Job drawing, mm, ordinate dimensions from the low corner. One solid piece. Give positions to 0.01 mm unless a question says otherwise; leave off trailing zeros. Order: outer loops, then holes, each group sorted by start corner. A loop starts at its lowest first (then second) coordinate and runs counter-clockwise, first axis right, second up. Notation, with made-up numbers: (5.5, 87.25) - (60.5, 87.25) arc R30 cw to (60.5, 126.25) - close; hole circle Ø4 at (62.5, 32.5). An arc over 180 degrees is marked (long way). One line per item, written item: value.
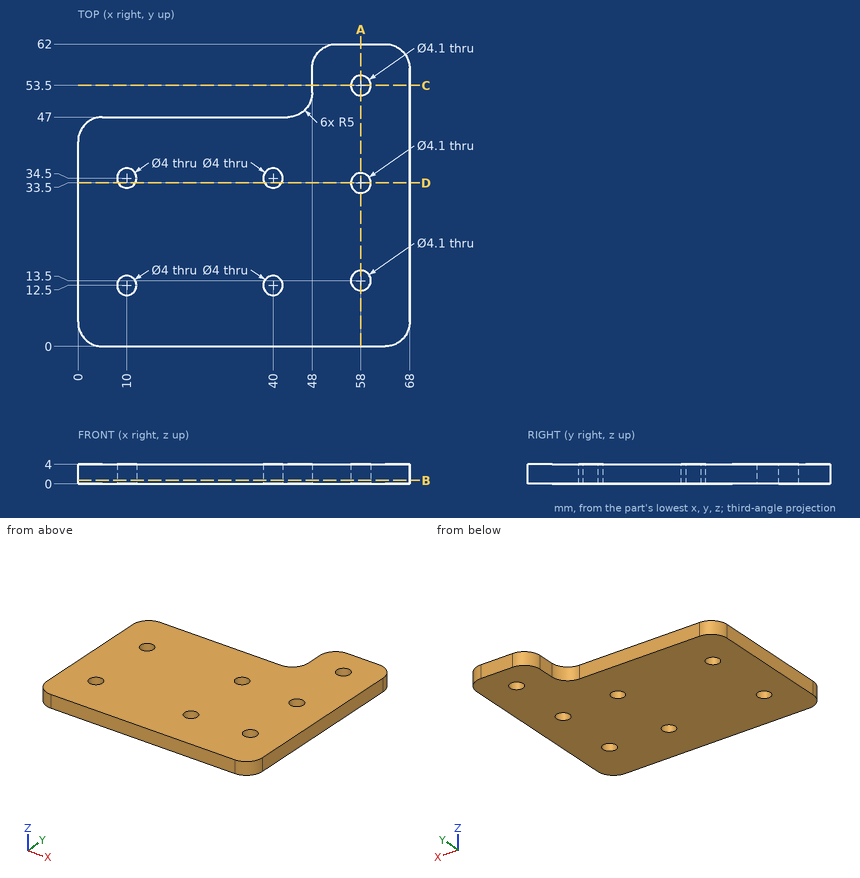
1) Slice it at B-B on z = 0.7. Write the cut outline in (x, y), then the cut area to 3 significant figures.
Answer:
outline: (0, 5) arc R5 ccw to (5, 0) - (63, 0) arc R5 ccw to (68, 5) - (68, 57) arc R5 ccw to (63, 62) - (53, 62) arc R5 ccw to (48, 57) - (48, 52) arc R5 cw to (43, 47) - (5, 47) arc R5 ccw to (0, 42) - close; hole circle Ø4 at (10, 12.5); hole circle Ø4 at (10, 34.5); hole circle Ø4 at (40, 12.5); hole circle Ø4 at (40, 34.5); hole circle Ø4.1 at (58, 13.5); hole circle Ø4.1 at (58, 33.5); hole circle Ø4.1 at (58, 53.5)
area: 3,380 mm2
2) Slice it at A-A on x = 58. Write the cut outline in (y, z), then the cut area to 3 significant figures.
Answer:
outline: (0, 0) - (11.45, 0) - (11.45, 4) - (0, 4) - close; (15.55, 0) - (31.45, 0) - (31.45, 4) - (15.55, 4) - close; (35.55, 0) - (51.45, 0) - (51.45, 4) - (35.55, 4) - close; (55.55, 0) - (62, 0) - (62, 4) - (55.55, 4) - close
area: 199 mm2
3) Wall check: line 1 along Y through (x, z) = (58, 2.1); line 2 along Y through (x, z) = (40, 0.9); line 3 along Y through (x, z) = (9.5, 2.25). Give the ranges that are in metal, low to high. Write a range as [from, to].
Answer:
line 1: y = [0, 11.45], [15.55, 31.45], [35.55, 51.45], [55.55, 62]
line 2: y = [0, 10.5], [14.5, 32.5], [36.5, 47]
line 3: y = [0, 10.56], [14.44, 32.56], [36.44, 47]
4) Drop flat-ended pins along their axis: P1, Ø2, axis at y = 10, z = 1, coming from the -X side; P2, Ø2, axis at x = 11.5, z = 1.5, coming from the +Y side; P3, Ø2, axis at y = 54.5, z = 1.5, coming from the -X side. Give the stop position or say it passes through.
Answer:
P1: stops at x = 0
P2: stops at y = 47
P3: stops at x = 48
5) Slice it at D-D on y = 33.5. Write the cut outline in (x, z).
Answer:
outline: (0, 0) - (8.27, 0) - (8.27, 4) - (0, 4) - close; (11.73, 0) - (38.27, 0) - (38.27, 4) - (11.73, 4) - close; (41.73, 0) - (55.95, 0) - (55.95, 4) - (41.73, 4) - close; (60.05, 0) - (68, 0) - (68, 4) - (60.05, 4) - close
6) Slice it at C-C on y = 53.5. Write the cut outline in (x, z).
Answer:
outline: (48, 0) - (55.95, 0) - (55.95, 4) - (48, 4) - close; (60.05, 0) - (68, 0) - (68, 4) - (60.05, 4) - close
